Could you check a few things on this drawing? It's one solid part, dimensions in mm from its lowest x, y, z. A direction names the side the tool comes from. Coordinates: 2 decimals unless noted, no trailing zeros. Write each loop counter-clockwise with the first axis right and the second up, starting at its lowest first coordinate (ties: lowest second). Pieces come first, ordered by that corner, then holes.
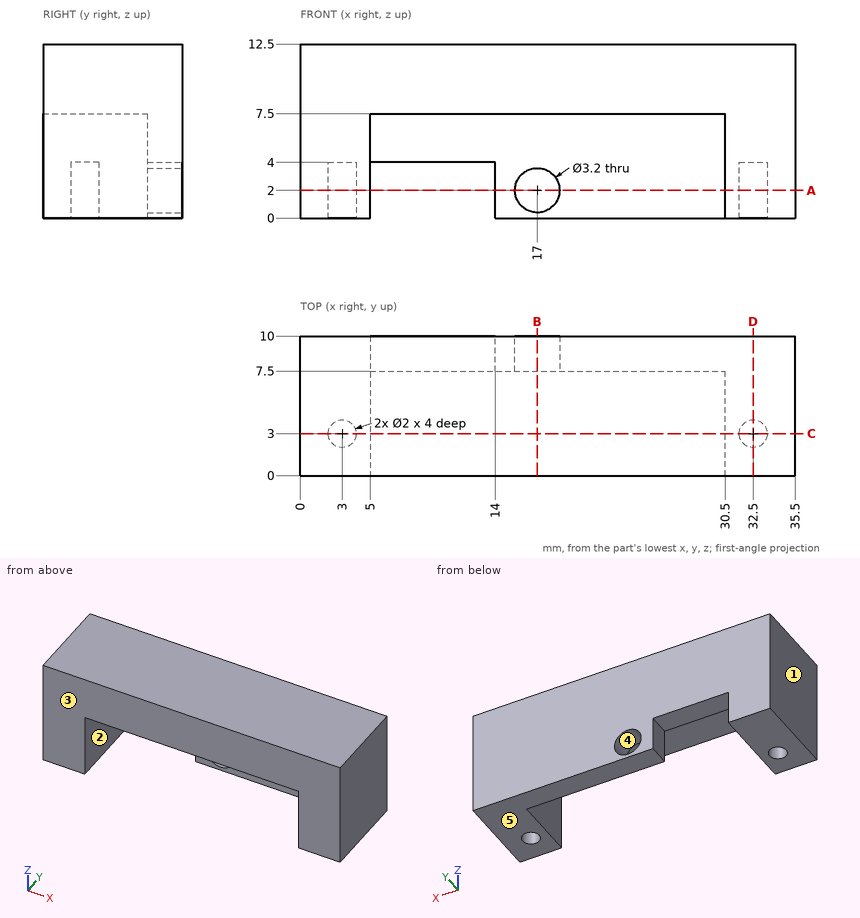
1) Imagine slicing it at B-B on x = 17. Please give me the cut outline in (y, z).
Values follow:
outline: (0, 7.5) - (7.5, 7.5) - (7.5, 3.6) - (10, 3.6) - (10, 12.5) - (0, 12.5) - close; (7.5, 0) - (10, 0) - (10, 0.4) - (7.5, 0.4) - close
2) We'd pull the mould along Z, two halves only. Please class the marked faces 3, 4 and 5: pulls with the +Z half, pulls with the -Z half, needs draft (parallel to the pull), parting line crosses it, or undercut.
Values follow:
face 3: needs draft
face 4: undercut
face 5: pulls with the -Z half
3) Imagine slicing it at D-D on x = 32.5. Please give me the cut outline in (y, z), then the cut area to 3 significant figures.
Values follow:
outline: (0, 0) - (2, 0) - (2, 4) - (4, 4) - (4, 0) - (10, 0) - (10, 12.5) - (0, 12.5) - close
area: 117 mm2
4) On a 3-axis mill with a long thin cutter (end or side, diameter ignored), from which of +Z, -Z, +X, -X, +Y, -Y can I reach the whole of each face in a straight line? I mean the marked faces 1 and 2. Say none if no direction works.
Values follow:
face 1: +Z, -Z, -X, +Y, -Y
face 2: -Z, -Y
5) I need wall thicknesses on probe 1 along X at (y, z) = (8.5, 2); probe 2 along X at (y, z) = (1.25, 4); probe 3 along Y at (x, z) = (3, 2.8). Which ranges of each line are inside material? Lowest first, please.
Values follow:
probe 1: x = 0 to 5, 14 to 15.4, 18.6 to 35.5
probe 2: x = 0 to 5, 30.5 to 35.5
probe 3: y = 0 to 2, 4 to 10
6) Imagine slicing it at C-C on y = 3. Please give me the cut outline in (x, z), then the cut area to 4 significant figures.
Values follow:
outline: (0, 0) - (2, 0) - (2, 4) - (4, 4) - (4, 0) - (5, 0) - (5, 7.5) - (30.5, 7.5) - (30.5, 0) - (31.5, 0) - (31.5, 4) - (33.5, 4) - (33.5, 0) - (35.5, 0) - (35.5, 12.5) - (0, 12.5) - close
area: 236.5 mm2
7) Imagine slicing it at A-A on z = 2. Please give me the cut outline in (x, y), then the cut area to 3 significant figures.
Values follow:
outline: (0, 0) - (5, 0) - (5, 10) - (0, 10) - close; (14, 7.5) - (15.4, 7.5) - (15.4, 10) - (14, 10) - close; (18.6, 7.5) - (30.5, 7.5) - (30.5, 0) - (35.5, 0) - (35.5, 10) - (18.6, 10) - close; hole circle Ø2 at (3, 3); hole circle Ø2 at (32.5, 3)
area: 127 mm2
8) Will these pins go through, and if not, where does the flat tip stop? pin 1 (2 mm diameter, centred on x = 13, z = 3.5, fed in from -Y); pin 2 (1.6 mm diameter, centred on x = 32.5, y = 3, fed in from -Z); pin 3 (2.5 mm diameter, centred on x = 17, z = 2, fed in from +Y); pin 4 (6 mm diameter, centred on x = 21, y = 4, fed in from -Z).
Values follow:
pin 1: stops at y = 7.5
pin 2: stops at z = 4
pin 3: passes through
pin 4: stops at z = 7.5
